Autodesk Fusion 360 part; units mm, degrees
sketch "Sketch1" plane through (0, 0, 0) normal (0, 0, 1) x (1, 0, 0)
  line L0 (-9.7956, 28.3971) -> (18.7794, 28.3971)
  line L1 (21.9544, 25.2221) -> (21.9544, -3.3529)
  line L2 (18.7794, -6.5279) -> (-9.7956, -6.5279)
  line L3 (-12.9706, -3.3529) -> (-12.9706, 25.2221)
  line L4 (-20.5581, 39.1596) -> (29.5419, 39.1596)
  line L5 (32.7169, 35.9846) -> (32.7169, -14.1154)
  line L6 (29.5419, -17.2904) -> (-20.5581, -17.2904)
  line L7 (-23.7331, -14.1154) -> (-23.7331, 35.9846)
  arc A0 (-20.5581, 39.1596) -> (-23.7331, 35.9846) centre (-20.5581, 35.9846) ccw
  arc A1 (-9.7956, 28.3971) -> (-12.9706, 25.2221) centre (-9.7956, 25.2221) ccw
  arc A2 (21.9544, 25.2221) -> (18.7794, 28.3971) centre (18.7794, 25.2221) ccw
  arc A3 (32.7169, 35.9846) -> (29.5419, 39.1596) centre (29.5419, 35.9846) ccw
  arc A4 (29.5419, -17.2904) -> (32.7169, -14.1154) centre (29.5419, -14.1154) ccw
  arc A5 (18.7794, -6.5279) -> (21.9544, -3.3529) centre (18.7794, -3.3529) ccw
  arc A6 (-12.9706, -3.3529) -> (-9.7956, -6.5279) centre (-9.7956, -3.3529) ccw
  arc A7 (-23.7331, -14.1154) -> (-20.5581, -17.2904) centre (-20.5581, -14.1154) ccw
  circle A8 centre (26.4057, -10.9792) radius 3
  line L8 (21.9544, 10.9346) -> (-12.9706, 10.9346)
  line L9 (4.4919, -6.5279) -> (4.4919, 28.3971)
  circle A9 centre (4.4919, -11.9091) radius 3
  line L10 (21.0245, -5.5979) -> (24.2844, -8.8579) construction
  line L11 (21.0245, -5.5979) -> (21.383, -5.5979) construction
  line L12 (31.787, -16.3604) -> (28.527, -13.1005) construction
  line L13 (31.787, -16.3604) -> (27.9277, -16.3604) construction
  circle A10 centre (26.4057, 32.8484) radius 3
  circle A11 centre (27.3356, 10.9346) radius 3
  circle A12 centre (-17.4219, 32.8484) radius 3
  circle A13 centre (4.4919, 33.7784) radius 3
  circle A14 centre (-17.4219, -10.9792) radius 3
  circle A15 centre (-18.3519, 10.9346) radius 3
  line L14 (-14.5581, 29.9846) -> (23.5419, 29.9846)
  line L15 (23.5419, 29.9846) -> (23.5419, -8.1154)
  line L16 (23.5419, -8.1154) -> (-14.5581, -8.1154)
  line L17 (-14.5581, -8.1154) -> (-14.5581, 29.9846)
  line L18 (4.4919, 29.9846) -> (4.4919, -8.1154)
  line L19 (23.5419, 10.9346) -> (-14.5581, 10.9346)
  point P0 (-12.9706, 28.3971)
  point P1 (21.9544, 28.3971)
  point P2 (-12.9706, -6.5279)
  point P3 (4.4919, 10.9346)
  point P4 (4.4919, 10.9346)
  dimension "d1" = 34.925
  dimension "d2" = 34.925
  dimension "d3" = 10.7625
  dimension "d4" = 10.7625
  dimension "d5" = 10.7625
  dimension "d6" = 10.7625
  dimension "d7" = 3.175
  dimension "d8" = 6
  dimension "d11" = 6
  dimension "d16" = 45
  dimension "d17" = 135
  dimension "d18" = 5.3813
  dimension "d20" = 360
  dimension "d25" = 38.1
  dimension "d26" = 38.1
extrude "Extrude1" add sketch "Sketch1" along normal blind 2 contours L0 L3 A1 L14 L17 L18 L19 | L0 L1 A2 L14 L15 L18 L19 | L2 L3 A6 L16 L17 L18 L19 | L1 L2 A5 L15 L16 L18 L19 | L4 L5 L6 L7 A0 A3 A4 A7 | A8 | A9 | A10 | A11 | A12 | A13 | A14 | A15
extrude "Extrude2" add sketch "Sketch1" against normal blind 2 contours L0 L3 A1 L14 L17 L18 L19 | L0 L1 A2 L14 L15 L18 L19 | L2 L3 A6 L16 L17 L18 L19 | L1 L2 A5 L15 L16 L18 L19 | L4 L5 L6 L7 A0 A3 A4 A7
sketch "Sketch2" plane through (0, 0, -2) normal (0, 0, -1) x (1, 0, 0)
  circle A0 centre (27.3356, -10.9346) radius 3
  circle A1 centre (26.4057, 10.9792) radius 3
  circle A2 centre (26.4057, -32.8484) radius 3
  circle A3 centre (-17.4219, 10.9792) radius 3
  circle A4 centre (-17.4219, -32.8484) radius 3
  circle A5 centre (4.4919, -33.7784) radius 3
  circle A6 centre (4.4919, 11.9091) radius 3
  arc A7 (-12.9706, -25.2221) -> (-9.7956, -28.3971) centre (-9.7956, -25.2221) ccw
  line L0 (-12.9706, -25.2221) -> (-12.9706, 3.3529)
  arc A8 (-9.7956, 6.5279) -> (-12.9706, 3.3529) centre (-9.7956, 3.3529) ccw
  line L1 (-9.7956, 6.5279) -> (18.7794, 6.5279)
  arc A9 (21.9544, 3.3529) -> (18.7794, 6.5279) centre (18.7794, 3.3529) ccw
  line L2 (21.9544, 3.3529) -> (21.9544, -25.2221)
  arc A10 (18.7794, -28.3971) -> (21.9544, -25.2221) centre (18.7794, -25.2221) ccw
  line L3 (18.7794, -28.3971) -> (-9.7956, -28.3971)
  circle A11 centre (-18.3519, -10.9346) radius 3
  arc A12 (-23.7331, -35.9846) -> (-20.5581, -39.1596) centre (-20.5581, -35.9846) ccw
  line L4 (-20.5581, -39.1596) -> (29.5419, -39.1596)
  arc A13 (29.5419, -39.1596) -> (32.7169, -35.9846) centre (29.5419, -35.9846) ccw
  line L5 (32.7169, -35.9846) -> (32.7169, 14.1154)
  arc A14 (32.7169, 14.1154) -> (29.5419, 17.2904) centre (29.5419, 14.1154) ccw
  line L6 (29.5419, 17.2904) -> (-20.5581, 17.2904)
  arc A15 (-20.5581, 17.2904) -> (-23.7331, 14.1154) centre (-20.5581, 14.1154) ccw
  line L7 (-23.7331, 14.1154) -> (-23.7331, -35.9846)
  line L8 (23.5419, 8.1154) -> (-14.5581, 8.1154)
  line L9 (-14.5581, 8.1154) -> (-14.5581, -29.9846)
  line L10 (-14.5581, -29.9846) -> (23.5419, -29.9846)
  line L11 (23.5419, -29.9846) -> (23.5419, 8.1154)
extrude "Extrude3" cut sketch "Sketch2" against normal blind 1.5875 contours L8 L9 L10 L11
equation "d1 = d25 - 0.125 in"
equation "d2 = d1"
equation "d3 = d8 + 0.1875 in"
equation "d4 = d3"
equation "d5 = d3"
equation "d6 = d3"
equation "d11 = d8"
equation "d14 = d6 / 2"
equation "d18 = d5 / 2"
equation "d26 = d25"
Could you check a few things on this model? Use its own coordinates, in mm. A direction names the side the tool comes from. Give positions to 0.01 mm unless a question says otherwise; leave off trailing zeros. Loops run counter-clockwise (first coordinate to the right, second up) from the corner with the lowest first, then second, coordinate; pieces in that order, holes last. Notation, with made-up numbers: (-21, 88) -> (-7, 88) arc R29 cw to (-7, 123) -> close; hole circle Ø9 at (61, 78.25). An arc over 180 degrees is marked (long way). Answer as CSV lines item,"result". Start each with the question number.
(1) I need wall thicknesses on probe 1 along X at (y, z) = (20, 1.75); probe 2 along Y at (x, z) = (-5, 1); probe 3 along X at (y, z) = (-4, -1.2). Which ranges of each line are inside material? Lowest first, please.
(2) If we section it at D-D on x = 25: Write out the boundary of the cut face in (y, z), then the cut area to 3 significant figures.
(3) If we section it at A-A on x = -1: Write out the boundary of the cut face in (y, z).
(4) Which directions (+Z, -Z, +X, -X, +Y, -Y) give clear straight access to the entire face, cutting with the end or side of a thin tool? Please do faces 4 (the cylindrical face through (-12.07, 27.44, 0.78)), 5 (the cylindrical face through (-21.35, 11.07, -0.99)), 6 (the flat face through (4, 39.16, 0)).
(5) If we section it at B-B on z = 1.4: Write out the boundary of the cut face in (x, y) (3 decimals).
(6) If we section it at C-C on y = 24: Write out the boundary of the cut face in (x, z), then the cut area to 3 significant figures.
(7) I'm going to push flat-ended pins straight in: pin 1 Ø5 at (x, y) = (4.49, 33.78) entering from -Z; pin 2 Ø8 at (x, y) = (-11.5, -7) entering from -Z. Where does each tip first touch, or does it pass through?
(8) We'd pull the mould along Y, two halves only. Please class faces 1 (the flat face through (4, 34, 0)), 2 (the cylindrical face through (-22.83, 38.2, -0.03)), 3 (the cylindrical face through (31.81, -16.34, -0.03)): released by +Y, released by -Y, zero draft, split by the parting line, or undercut.
Computed:
1,probe 1,"x = -23.73 to -12.97, 21.95 to 32.72"
1,probe 2,"y = -17.29 to -6.53, 28.4 to 39.16"
1,probe 3,"x = -23.73 to -14.56, 23.54 to 32.72"
2,outline,"(-17.29, -2) -> (-13.63, -2) -> (-13.63, 0) -> (-8.33, 0) -> (-8.33, -2) -> (9.05, -2) -> (9.05, 0) -> (12.82, 0) -> (12.82, -2) -> (30.2, -2) -> (30.2, 0) -> (35.5, 0) -> (35.5, -2) -> (39.16, -2) -> (39.16, 2) -> (-17.29, 2) -> close"
2,area,"197 mm2"
3,outline,"(-17.29, -2) -> (-8.12, -2) -> (-8.12, -0.41) -> (-6.53, -0.41) -> (-6.53, 2) -> (-17.29, 2) -> close; (28.4, -0.41) -> (29.98, -0.41) -> (29.98, -2) -> (39.16, -2) -> (39.16, 2) -> (28.4, 2) -> close"
4,face 4,"+Z, -Z"
4,face 5,"-Z"
4,face 6,"+Z, -Z, +X, -X, +Y"
5,outline,"(-23.733, -14.115) arc R3.175 ccw to (-20.558, -17.29) -> (29.542, -17.29) arc R3.175 ccw to (32.717, -14.115) -> (32.717, 35.985) arc R3.175 ccw to (29.542, 39.16) -> (-20.558, 39.16) arc R3.175 ccw to (-23.733, 35.985) -> close; hole (-12.971, -3.353) arc R3.175 ccw to (-9.796, -6.528) -> (18.779, -6.528) arc R3.175 ccw to (21.954, -3.353) -> (21.954, 25.222) arc R3.175 ccw to (18.779, 28.397) -> (-9.796, 28.397) arc R3.175 ccw to (-12.971, 25.222) -> close"
6,outline,"(-23.73, -2) -> (-14.56, -2) -> (-14.56, -0.41) -> (-12.97, -0.41) -> (-12.97, 2) -> (-23.73, 2) -> close; (21.95, -0.41) -> (23.54, -0.41) -> (23.54, -2) -> (32.72, -2) -> (32.72, 2) -> (21.95, 2) -> close"
6,area,"81.1 mm2"
7,pin 1,"stops at z = 0"
7,pin 2,"stops at z = -2"
8,face 1,"undercut"
8,face 2,"released by +Y"
8,face 3,"released by -Y"
